Geometry check sheet. Reference: the model listing, model coordinates, mm. Face numbers are marked on the shaded views. A direction names the side the tool comes from. Round coordinates to 2 decimals unless told otherwise and drop trailing zeros. Write each loop counter-clockwise with the first axis right and the second up, starting at its lowest first coordinate (ties: lowest second). Pieces come first, ordered by that corner, then holes. Notation, with made-up numbers: (64, -23) -> (75, -23) arc R15 ccw to (75, 6) -> close; hole circle Ø7 at (47, -14). An arc over 180 degrees is marked (long way). Return JSON: item names as keys, results as strings. Group by question number.
from build123d import *

# Parameters (mm, degrees)
SKETCH2_R           = 2
BOSS_EXTRUDE2_DEPTH = 3
SKETCH3_R           = 2
BOSS_EXTRUDE3_DEPTH = 20
BOSS_EXTRUDE4_DEPTH = 3


with BuildPart() as part:
    # Sketch2 → Boss-Extrude2 (new body)
    with BuildSketch(Plane.XY):
        Polygon((0, 4.618802154), (-4, 2.309401077), (-4, -2.309401077), (0, -4.618802154), (4, -2.309401077), (4, 2.309401077), align=None)
        Circle(SKETCH2_R, mode=Mode.SUBTRACT)
    extrude(amount=BOSS_EXTRUDE2_DEPTH)

    # Sketch3 → Boss-Extrude3 (add)
    with BuildSketch(Plane(origin=(2, 3.464101615, 0), x_dir=(0.8660254037844386, -0.4999999999999999, 0), z_dir=(0.49999999999999994, 0.8660254037844387, 0))):
        with Locations(Location((0, -1.5, 0), (0, 0, 48.590377891))):
            Circle(SKETCH3_R)
    extrude(amount=BOSS_EXTRUDE3_DEPTH)

    # Sketch4 → Boss-Extrude4 (add)
    with BuildSketch(Plane(origin=(7.5, 12.990381057, 0), x_dir=(0.8660254037844386, -0.4999999999999999, 0), z_dir=(0.49999999999999994, 0.8660254037844387, 0))):
        Polygon((0.885290866, 3.033165937), (-3.483191429, 1.533267348), (-4.368482294, -2.999898589), (-0.885290866, -6.033165937), (3.483191429, -4.533267348), (4.368482294, -0.000101411), align=None)
    extrude(amount=BOSS_EXTRUDE4_DEPTH)


solid = part.part
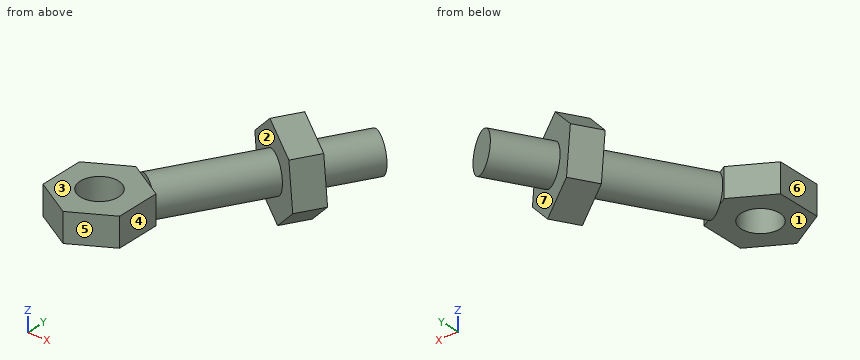
1) Material ranges on probe 1 along X at (y, z) = (-2.25, 2.25); probe 2 along Z at (x, y) = (2, -3); probe 3 along Y at (x, z) = (11.75, 0.5), recorded low to high. Write a range as [from, to].
2) Sectioned sample at C-C on z = 1.5. Enter the section's corners in (x, y).
3) Sectioned sample at B-B on x = -0.75. Enter the section's corners in (y, z), and give its area (3 significant figures).
4) Sectioned sample at A-A on y = 0. Enter the section's corners in (x, z).
5) Go/stop test with flat-tipped pins: P1, Ø6.5, axis at x = -1, y = 2, coming from the -Z side; P2, Ø4, axis at x = -1.5, y = -2, coming from the +Z side; P3, Ø4, axis at x = 4.5, y = 2, coming from the -Z side. Record where each tip stops, or that it passes through.
6) Tool access check on the marked faces 1, 2, 3 and 4. Record the directions out of +Z, -Z, +X, -X, +Y, -Y that give a thin tool (end or side, any length) a straight path to the whole face; none if there is none.
7) Mould release check, pull along X, two halves, no side actions. Record for the marked faces 5, 6 and 7: +X half, -X half, draft (parallel to the pull), parting line (faces both ways), or undercut.
8) Sectioned sample at D-D on z = 5. Enter the section's corners in (x, y).
Evaluation:
{
 "1": {"probe 1": "x = [-4, 4]", "probe 2": "z = [0, 3]", "probe 3": "y = [11.81, 14], [16.89, 20.93]"},
 "2": {"outline": "(-4, -2.31) -> (0, -4.62) -> (4, -2.31) -> (4, 2.31) -> (3.73, 2.46) -> (9.23, 11.99) -> (11.03, 10.95) -> (12.53, 13.55) -> (10.73, 14.59) -> (13.73, 19.78) -> (10.27, 21.78) -> (7.27, 16.59) -> (5.47, 17.63) -> (3.97, 15.03) -> (5.77, 13.99) -> (0.27, 4.46) -> (0, 4.62) -> (-4, 2.31) -> close; hole circle Ø4 at (0, 0)"},
 "3": {"outline": "(-4.19, 0) -> (-1.85, 0) -> (-1.85, 3) -> (-4.19, 3) -> close; (1.85, 0) -> (4.19, 0) -> (4.19, 3) -> (1.85, 3) -> close", "area": "14.0 mm2"},
 "4": {"outline": "(-4, 0) -> (-2, 0) -> (-2, 3) -> (-4, 3) -> close; (2, 0) -> (4, 0) -> (4, 3) -> (2, 3) -> close"},
 "5": {"P1": "stops at z = -0.49", "P2": "stops at z = 3", "P3": "stops at z = -0.29"},
 "6": {"face 1": "-Z, -X, -Y", "face 2": "none", "face 3": "+Z, -X, -Y", "face 4": "+Z, -Z, +X, -Y"},
 "7": {"face 5": "+X half", "face 6": "-X half", "face 7": "undercut"},
 "8": {"outline": "(5.71, 14.03) -> (9.34, 11.93) -> (10.84, 14.53) -> (7.21, 16.62) -> close"}
}
